Geometry check sheet. Reference: the model listing, model coordinates, mm. A direction names the side the tool comes from. Coordinates: 2 decimals unless noted, no trailing zeros. Order: outer loops, then holes, each group sorted by start corner. A loop starts at its lowest first (then second) coordinate and runs counter-clockwise, first axis right, second up. Notation, with made-up numbers: (29.25, 17) - (80.25, 17) arc R17 ccw to (80.25, 47) - close; hole circle Ø10 at (-19, 45.25). An arc over 180 degrees is marked (long way). One line per item, written item: value. Start each with the question number.
```python
from build123d import *

# Parameters (mm, degrees)
PAD_DEPTH    = 2
PAD001_DEPTH = 2


with BuildPart() as pad001:
    # Sketch → Pad (new body)
    with BuildSketch(Plane.XY):
        with BuildLine():
            Line((60, 8), (60, 82.000001))
            ThreePointArc((60, 82.000001), (58.434586, 89.869877), (53.976662, 96.541638))
            Line((40.541631, 109.976664), (53.976662, 96.541638))
            ThreePointArc((40.541631, 109.976664), (33.869872, 114.434584), (25.999999, 115.999997))
            Line((7.999999, 115.999997), (25.999999, 115.999997))
            ThreePointArc((7.999999, 115.999997), (2.343146, 113.656851), (0, 107.999998))
            Line((0, 107.999998), (0, 8))
            ThreePointArc((0, 8), (2.343146, 2.343146), (8, 0))
            Line((8, 0), (52, 0))
            ThreePointArc((52, 0), (57.656854, 2.343146), (60, 8))
        make_face()
    extrude(amount=PAD_DEPTH)

    # Sketch001 → Pad001 (new body)
    with BuildSketch(Plane.XY.offset(2)):
        with BuildLine():
            ThreePointArc((8.00001, 113.999998), (3.757363, 112.242642), (2, 107.999998))
            Line((2, 107.999998), (2, 8))
            ThreePointArc((2, 8), (3.757359, 3.757359), (8, 2))
            Line((8, 2), (52, 2))
            ThreePointArc((52, 2), (56.242642, 3.757359), (58.000001, 8))
            Line((58.000001, 82), (58.000001, 8))
            ThreePointArc((58.000001, 82), (56.586824, 89.104519), (52.562435, 95.127438))
            Line((39.127419, 108.562437), (52.562435, 95.127438))
            ThreePointArc((39.127419, 108.562437), (33.104503, 112.586822), (25.99999, 113.999998))
            Line((8.00001, 113.999998), (25.99999, 113.999998))
        make_face()
    extrude(amount=PAD001_DEPTH)


with BuildPart() as part_mirroring:
    # Part__Mirroring: instance of Pad001
    add(pad001.part.mirror(Plane(origin=(0, 0, 0), x_dir=(0, 1, 0), z_dir=(0, 0, 1))))


solid = part_mirroring.part
```
Q1. Gauge pin test, flat ends, axial feed: P1, Ø1.5, axis at x = 26.5, z = -1.5, coming from the +Y side; P2, Ø0.6, axis at x = 16, z = -3, coming from the +Y side. Record the tip position at first contact, or that the pin passes through.
Q2. Cross-section at B-B, the plane y = 75.5. Enter the section's corners in (x, z).
Q3. Cross-section at A-A, the plane z = -1. Enter the section's corners in (x, y) (3 decimals), and give its area (3 significant figures).
Q4. Material ranges on probe 1 along X at (y, z) = (56, -2.35); probe 2 along Y at (x, z) = (25.5, -2.4); probe 3 along X at (y, z) = (85.5, -1.7), recorded low to high.
Q5. Cross-section at C-C, the plane x = 19.5. Enter the section's corners in (y, z), and give its area (3 significant figures).
Q6. Set-up check for faces 1 (the flat face through (17, 114, -3)), 2 (the cylindrical face through (56.196, 3.711, -2.986)), 3 (the cylindrical face through (56.626, 89.01, -2.986)), 4 (the flat face through (2, 59, -3)): record each of +Z, -Z, +X, -X, +Y, -Y from which the full face is reachable in a straight line by a thin tool's end or side.
Check result:
1. P1: stops at y = 116
1. P2: stops at y = 114
2. outline: (0, -2) - (2, -2) - (2, -4) - (58, -4) - (58, -2) - (60, -2) - (60, 0) - (0, 0) - close
3. outline: (0, 8) arc R8 ccw to (8, 0) - (52, 0) arc R8 ccw to (60, 8) - (60, 82) arc R20.565 ccw to (53.977, 96.542) - (40.542, 109.977) arc R20.565 ccw to (26, 116) - (8, 116) arc R8 ccw to (0, 108) - close
3. area: 6,580 mm2
4. probe 1: x = 2 to 58
4. probe 2: y = 2 to 114
4. probe 3: x = 0 to 59.7
5. outline: (0, -2) - (2, -2) - (2, -4) - (114, -4) - (114, -2) - (116, -2) - (116, 0) - (0, 0) - close
5. area: 456 mm2
6. face 1: -Z, +X, -X, +Y
6. face 2: -Z, +X, -Y
6. face 3: -Z, +X, +Y
6. face 4: -Z, -X, +Y, -Y
